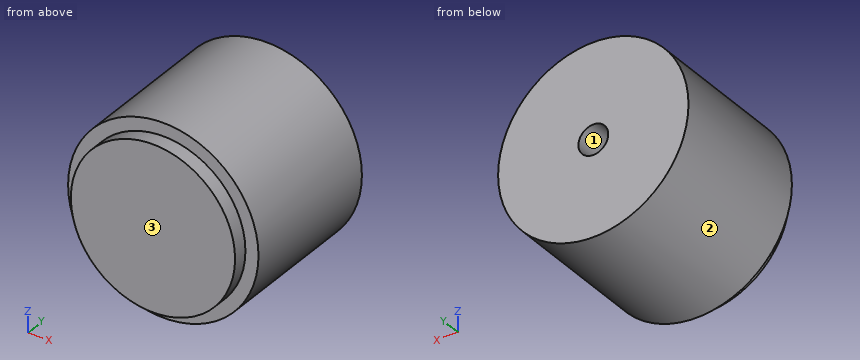
Autodesk Inventor part; units mm, degrees
ref_plane "YZ Plane" through (0, 0, 0) normal (1, 0, 0) x (0, 1, 0)
ref_plane "XZ Plane" through (0, 0, 0) normal (0, 1, 0) x (-1, 0, 0)
ref_plane "XY Plane" through (0, 0, 0) normal (0, 0, 1) x (1, 0, 0)
sketch "Sketch1" plane through (0, 0, 0) normal (0, 1, 0) x (-1, 0, 0)
  circle A0 centre (0, 0) radius 12.75
  dimension "d0" = 25.5
extrude "Extrusion1" add sketch "Sketch1" along normal blind 20
sketch "Sketch2" plane through (0, 0, 0) normal (0, -1, 0) x (1, 0, 0)
  circle A0 centre (0, 0) radius 11
  dimension "d3" = 22
extrude "Extrusion2" add sketch "Sketch2" along normal blind 2
sketch "Sketch3" plane through (0, 20, 0) normal (0, 1, 0) x (1, 0, 0)
  point P0 (0, 0)
  point P1 (0, 0)
hole "Hole1" at (0, 20, 0) direction (0, -1, 0) diameter 4 depth 5
thread "Thread1"
properties part number "magnet"
Geometry check sheet. Reference: the model listing, model coordinates, mm. Face numbers are marked on the shaded views. Round coordinates to 2 decimals unless told otherwise and drop trailing zeros. Order: outer loops, then holes, each group sorted by start corner. A loop starts at its lowest first (then second) coordinate and runs counter-clockwise, first axis right, second up. Notation, with made-up numbers: M 48,66.5 L 107,66.5 A18 cw 107,73.5 Z; hole C 69,16.5 d9. An arc over 180 degrees is marked long. Answer in a Markdown table with one row per item. Add a question column.
Item 1: Sectioned sample at D-D, the plane y = 6.5. Enter the section's corners in (x, z), plus the area to 3 significant figures.
Item 2: Sectioned sample at A-A, the plane z = 0. Enter the section's corners in (x, y).
Item 3: Sectioned sample at B-B, the plane x = 0. Enter the section's corners in (y, z), plus the area to 3 significant figures.
Item 4: Draft check along X on the marked faces 1, 2 and 3. Enter one of: released by +X, released by -X, zero draft, split by the parting line, or undercut.
Item 5: Sectioned sample at C-C, the plane y = 18.75. Enter the section's corners in (x, z).
Item 6: Depth check by flat-ended pin: pin 1 Ø1.5 at (x, y) = (-6.5, 3.5) entering from +Z; pin 2 Ø5 at (x, y) = (-2.5, 15.5) entering from +Z; pin 3 Ø2.5 at (x, z) = (0, 0) entering from +Y; pin 4 Ø2 at (y, z) = (17.5, -9) entering from -X. Enter the tip coordinate at first touch or a pass-through.
Item 7: Material ranges on L1, parallel to Z at x = 0, y = 18.25; L2, parallel to Y at x = -8, z = 8.5; L3, parallel to Y at x = 1.5, z = 0.5, recorded low to high. Write a range as [from, to].
Filled in:
| question | item | result |
|---|---|---|
| 1 | outline | C 0,0 d25.5 |
| 1 | area | 511 mm² |
| 2 | outline | M -12.75,0 L -11,0 L -11,-2 L 11,-2 L 11,0 L 12.75,0 L 12.75,20 L 2,20 L 2,15 L -2,15 L -2,20 L -12.75,20 Z |
| 3 | outline | M -2,-11 L 0,-11 L 0,-12.75 L 20,-12.75 L 20,-2 L 15,-2 L 15,2 L 20,2 L 20,12.75 L 0,12.75 L 0,11 L -2,11 Z |
| 3 | area | 534 mm² |
| 4 | face 1 | undercut |
| 4 | face 2 | split by the parting line |
| 4 | face 3 | zero draft |
| 5 | outline | C 0,0 d25.5; hole C 0,0 d4 |
| 6 | pin 1 | stops at z = 11.38 |
| 6 | pin 2 | stops at z = 12.75 |
| 6 | pin 3 | stops at y = 15 |
| 6 | pin 4 | stops at x = -9.93 |
| 7 | L1 | z = [-12.75, -2], [2, 12.75] |
| 7 | L2 | y = [0, 20] |
| 7 | L3 | y = [-2, 15] |
